Read the model definition and answer for the solid it produces. Units are mm, in the model's axes. A direction names the side the tool comes from. Coordinates: 2 decimals unless noted, no trailing zeros. Order: outer loops, then holes, each group sorted by start corner. A loop starts at its lowest first (then second) coordinate and runs counter-clockwise, first axis right, second up. Notation, with made-up numbers: (55.5, -12) - (67.5, -12) arc R32 ccw to (67.5, 16) - close; hole circle Ø7 at (58.25, 45.25). An arc over 180 degrees is marked (long way). Write item = value, one per line.
from build123d import *

# Parameters (mm, degrees)
SKETCH2_R          = 2
CUT_EXTRUDE1_DEPTH = 4.81


with BuildPart() as part:
    # Sketch1 → Revolve1 (revolve)
    with BuildSketch(Plane.XY):
        Polygon((0, 0.6), (3.5, 0.6), (3.5, 0), (5.5, 0), (6.914213562, 1.414213562), (6.914213562, 2.475397075), (3.556, 2.475397075), (3.556, 4.41), (0, 4.41), align=None)
    revolve(axis=Axis((0, 4.41, 0), (0, -1, 0)))

    # Sketch2 → Cut-Extrude1 (cut, through all)
    with BuildSketch(Plane.XZ.offset(-0.6)):
        Circle(SKETCH2_R)
    extrude(amount=-CUT_EXTRUDE1_DEPTH, mode=Mode.SUBTRACT)


solid = part.part
1) Flat-ended cylindrical pins translate along their axes: pin 1 Ø1 at (y, z) = (2.5, -2) entering from -X; pin 2 Ø1 at (y, z) = (1.5, -1) entering from -X. Find the tip coordinate at first contact, or state that the pin passes through.
Returned:
pin_1 = -6.75
pin_2 = -6.9
2) The part is cut by section B-B (z = 0). Determine the outline of the cut face in (x, y).
Returned:
outline = (-6.91, 1.41) - (-5.5, 0) - (-3.5, 0) - (-3.5, 0.6) - (-2, 0.6) - (-2, 4.41) - (-3.56, 4.41) - (-3.56, 2.48) - (-6.91, 2.48) - close; (2, 0.6) - (3.5, 0.6) - (3.5, 0) - (5.5, 0) - (6.91, 1.41) - (6.91, 2.48) - (3.56, 2.48) - (3.56, 4.41) - (2, 4.41) - close
3) Determine the mould class of faces 1 (the face through (-0.77, 3.46, -3.47)), 2 (the face through (-4, 0, 0)), 3 (the face through (0, 2, -2)) for opening direction X: pulls with the +X half, pulls with the -X half, needs draft (parallel to the pull), parting line crosses it, or undercut.
Returned:
face_1 = parting line crosses it
face_2 = needs draft
face_3 = undercut
4) Straight lines are drawn through the part: line 1 along Z through (x, y) = (0, 1.8); line 2 along Z through (x, y) = (1.5, 0.35); line 3 along X through (y, z) = (2.65, -1.25). For each, find the intervals that lie inside material, in ascending order. Write a range as from..to.
Returned:
line_1 = -6.91..-2, 2..6.91
line_2 = -5.65..-3.16, 3.16..5.65
line_3 = -3.33..-1.56, 1.56..3.33
5) The part is cut by section A-A (x = 0). Determine the outline of the cut face in (y, z).
Returned:
outline = (0, -5.5) - (1.41, -6.91) - (2.48, -6.91) - (2.48, -3.56) - (4.41, -3.56) - (4.41, -2) - (0.6, -2) - (0.6, -3.5) - (0, -3.5) - close; (0, 3.5) - (0.6, 3.5) - (0.6, 2) - (4.41, 2) - (4.41, 3.56) - (2.48, 3.56) - (2.48, 6.91) - (1.41, 6.91) - (0, 5.5) - close
6) For faces 4 (the face through (3.233, 0.296, -1.341)), 5 (the face through (-5.487, 1.952, -4.207)), 6 (the face through (3, 2.475, -3)), determine the directions among +Z, -Z, +X, -X, +Y, -Y from which every point of the face is accessible in a straight line to the end or side of a thin tool.
Returned:
face_4 = -Y
face_5 = +Y, -Y
face_6 = +Y
